from build123d import *

# Parameters (mm, degrees)
SKETCH_W         = 70
SKETCH_H         = 50
SKETCH001_W      = 55
SKETCH001_H      = 35
SKETCH002_R      = 9
POCKET_DEPTH     = 30
HOLE_D           = 5
HOLE_CBORE_D     = 10
HOLE_CBORE_DEPTH = 18
FILLET_R         = 3


with BuildPart() as part:
    # Sketch → AdditiveLoft section 0
    with BuildSketch(Plane.XY):
        Rectangle(SKETCH_W, SKETCH_H)
    # Sketch001 (on DatumPlane) → AdditiveLoft section 1
    with BuildSketch(Plane.XY.offset(30)):
        Rectangle(SKETCH001_W, SKETCH001_H)
    loft()

    # Sketch002 (on DatumPlane) → Pocket (cut)
    with BuildSketch(Plane.XY.offset(30)):
        Circle(SKETCH002_R)
    extrude(amount=-POCKET_DEPTH, mode=Mode.SUBTRACT)

    # Hole (through all)
    with Locations(Plane.XY.offset(30)):
        with Locations((-20, 0), (20, 0)):
            CounterBoreHole(HOLE_D / 2, HOLE_CBORE_D / 2, HOLE_CBORE_DEPTH)

    # Fillet
    fillet_edges = [part.edges().sort_by_distance(p)[0] for p in [
        (-31.25, -21.25, 15),
        (0, -17.5, 30),
        (-27.5, 0, 30),
        (31.25, -21.25, 15),
        (27.5, 0, 30),
        (0, 17.5, 30),
        (-31.25, 21.25, 15),
        (31.25, 21.25, 15),
    ]]
    fillet(fillet_edges, radius=FILLET_R)


solid = part.part
CAD build for the part. Positions are in the model's coordinates, mm. A direction names the side the tool comes from. Coordinates: 2 decimals unless noted, no trailing zeros. Use a Markdown table: item, result. Add a question column.
Item 1: Drill centre lines: L1, parallel to Z at x = -22, y = 2; L2, parallel to X at y = -1, z = 4; L3, parallel to Y at x = -3, z = 17. Where is each one in solid material? Low to high. Write a range as from..to.
Item 2: 3-axis set-ups, long thin cutter, end or side, ignore diameter. For faces 4 (the face through (-25, 0, 21)), 5 (the face through (-17.5, 0.1, 5.9)): which of +Z, -Z, +X, -X, +Y, -Y reach the whole face in a straight line?
Item 3: Flat gauge pins, fed straight in: pin 1 (11 mm diameter, centred on x = 0, y = 0, fed in from +Z); pin 2 (1 mm diameter, centred on x = -15.5, y = -15.5, fed in from -Z); pin 3 (5 mm diameter, centred on y = -6, z = 23, fed in from -X) (3 decimals); pin 4 (12 mm diameter, centred on x = 11, z = 12.5, fed in from +Y) (3 decimals). Where does each tip first touch, or does it go through?
Item 4: Mould opens along Y. For faces 1 (the face through (22, -2, 12)), 2 (the face through (5, -8, 30)), 3 (the face through (22.5, 0.1, 5.9)) say: pulls with the +Y half, pulls with the -Y half, needs draft (parallel to the pull), parting line crosses it, or undercut.
Item 5: Band-saw the part on A-A, the plane y = 0. Give the number of separate pieces and of enclosed holes in the cut face, and give its area (3 significant figures).
Numbers:
| question | item | result |
|---|---|---|
| 1 | L1 | 0..12 |
| 1 | L2 | -34..-22.29, -17.71..-8.94, 8.94..17.71, 22.29..34 |
| 1 | L3 | -20.75..-8.49, 8.49..20.75 |
| 2 | face 4 | +Z |
| 2 | face 5 | +Z, -Z |
| 3 | pin 1 | through |
| 3 | pin 2 | z = 0 |
| 3 | pin 3 | x = -29.875 |
| 3 | pin 4 | y = 23.375 |
| 4 | face 1 | undercut |
| 4 | face 2 | needs draft |
| 4 | face 3 | undercut |
| 5 | separate pieces | 4 |
| 5 | enclosed holes | 0 |
| 5 | area | 853 mm2 |
